The model under review builds one solid part; all positions refer to its coordinate system, in mm. A direction names the side the tool comes from. Round coordinates to 2 decimals unless told otherwise and drop trailing zeros. Write each loop counter-clockwise with the first axis right and the second up, starting at its lowest first coordinate (ties: lowest second). Pieces come first, ordered by that corner, then holes. Notation, with made-up numbers: (67, 23) -> (86, 23) arc R32 ccw to (86, 57) -> close; hole circle Ø10 at (67.25, 12). An arc over 180 degrees is marked (long way). Use CSV: the item, a comma, the result in double quotes. Start each with the question number.
1) Wall thickness on probe 1 along X at (y, z) = (33, 3); probe 2 along Y at (x, z) = (-45, 5); probe 3 along Z at (x, y) = (-44, 21.5): over which ranges is each line inside the solid? List them lowest first. Write a range as [from, to].
2) Mouldability with a two-part tool opening along X and no side actions: class faces 3 (the face through (-35, 2.092, 19)), 4 (the face through (-21.96, 26.74, 42.4)), 5 (the face through (-14.63, 27, 12)) as released by +X, released by -X, zero draft, split by the parting line, or undercut.
3) Machinability: for faces 1 (the face through (-54.63, 27, 12)), 2 (the face through (-59.63, 27, 17)), which of the approach directions +Z, -Z, +X, -X, +Y, -Y give a long, thin tool a straight path to every point of the face, cutting with its end or side? Answer none if there is none.
4) For pin 1 Ø4 at (x, y) = (-33, 8.5) entering from +Z; pin 2 Ø6 at (x, y) = (-40, 17.5) entering from +Z, all flat-tipped, find the tip position at first contact; note any pin that passes through.
5) Take a section at A-A, the plane z = 10. Give the boundary of the cut face in (x, y), then the cut area to 3 significant figures.
6) Take a section at C-C, the plane x = -31. Give the boundary of the cut face in (y, z).
7) Take a section at D-D, the plane x = -42. Give the boundary of the cut face in (y, z).
from build123d import *

# Parameters (mm, degrees)
F0_W     = 50
F0_H     = 50
F0_W_2   = 40
F0_H_2   = 40
F1_DEPTH = 25
F2_W     = 50
F2_H     = 50
F3_DEPTH = 25
F4_SIZE2 = 14.99999
F4_SIZE  = 24.99999


# Not quite as in the source:
# - a fillet or chamfer is up to 0.001 mm smaller than in the source, because OpenCascade refuses the exact size


with BuildPart() as f1:
    # F0 (on Top) → F1 (new body)
    with BuildSketch(Plane.XY):
        with Locations((-34.6303719711, 27.0920880139)):
            Rectangle(F0_W, F0_H)
        with Locations((-34.6303719711, 27.0920880139)):
            Rectangle(F0_W_2, F0_H_2, mode=Mode.SUBTRACT)
    extrude(amount=F1_DEPTH)

    # F2 (on face) → F3 (join)
    with BuildSketch(Plane.XY.offset(25)):
        with Locations((-34.6303719711, 27.0920880139)):
            Rectangle(F2_W, F2_H)
    extrude(amount=F3_DEPTH)

    # F4 (size 25 and 15 in the source; OpenCascade refuses exactly that, so slightly less here)
    f4_edges = [f1.edges().sort_by_distance(p)[0] for p in [
        (-59.630372, 27.092088, 50),
        (-9.630372, 27.092088, 50),
    ]]
    f4_side = f1.faces().sort_by_distance((-34.630372, 27.092088, 50))[0]
    chamfer(f4_edges, length=F4_SIZE, length2=F4_SIZE2, reference=f4_side)


solid = f1.part
Values found:
1,probe 1,"[-59.63, -54.63], [-14.63, -9.63]"
1,probe 2,"[2.09, 7.09], [47.09, 52.09]"
1,probe 3,"[25, 44.38]"
2,face 3,"zero draft"
2,face 4,"released by +X"
2,face 5,"undercut"
3,face 1,"-Z"
3,face 2,"+Z, -Z, -X, +Y, -Y"
4,pin 1,"z = 50"
4,pin 2,"z = 48.58"
5,outline,"(-59.63, 2.09) -> (-9.63, 2.09) -> (-9.63, 52.09) -> (-59.63, 52.09) -> close; hole (-54.63, 7.09) -> (-14.63, 7.09) -> (-14.63, 47.09) -> (-54.63, 47.09) -> close"
5,area,"900 mm²"
6,outline,"(2.09, 0) -> (7.09, 0) -> (7.09, 25) -> (47.09, 25) -> (47.09, 0) -> (52.09, 0) -> (52.09, 47.82) -> (2.09, 47.82) -> close"
7,outline,"(2.09, 0) -> (7.09, 0) -> (7.09, 25) -> (47.09, 25) -> (47.09, 0) -> (52.09, 0) -> (52.09, 45.58) -> (2.09, 45.58) -> close"
